from build123d import *

# Parameters (mm, degrees)
SKETCH1_R                                         = 16.7
SKETCH1_R_2                                       = 12.7
BOSS_EXTRUDE1_DEPTH                               = 10
SKETCH2_W                                         = 22.16607393
SKETCH2_H                                         = 10
SKETCH2_W_2                                       = 4
SKETCH2_H_2                                       = 30
BOSS_EXTRUDE2_DEPTH                               = 10
SKETCH4_W                                         = 8
SKETCH4_H                                         = 11.78611706
BOSS_EXTRUDE3_DEPTH                               = 10
FILLET3_R                                         = 1
CSK_FOR_6_FLAT_HEAD_MACHINE_SCREW_100_D           = 4.3053
CSK_FOR_6_FLAT_HEAD_MACHINE_SCREW_100_CSINK_D     = 7.0866
CSK_FOR_6_FLAT_HEAD_MACHINE_SCREW_100_CSINK_ANGLE = 100
INTERSECT3_START                                  = -42.1
INTERSECT3_OUTLINE_R                              = 2.15265
INTERSECT3_DEPTH                                  = 42.1


# Read off the part's stored shape, not the designer's step: CSK for #4 Flat Head Machine Screw (100)1, Intersect3
with BuildPart() as part:
    # Sketch1 → Boss-Extrude1 (new body)
    with BuildSketch(Plane.XY):
        Circle(SKETCH1_R)
        Circle(SKETCH1_R_2, mode=Mode.SUBTRACT)
    extrude(amount=BOSS_EXTRUDE1_DEPTH)

    # Sketch2 → Boss-Extrude2 (add)
    with BuildSketch(Plane(origin=(0, 0, 0), x_dir=(-1, 0, 0), z_dir=(0, 0, -1))):
        with Locations((27.016963035, 0)):
            Rectangle(SKETCH2_W, SKETCH2_H)
        with Locations((40.1, 0)):
            Rectangle(SKETCH2_W_2, SKETCH2_H_2)
    extrude(amount=-BOSS_EXTRUDE2_DEPTH)

    # Sketch4 → Boss-Extrude3 (add)
    with BuildSketch(Plane(origin=(0, 0, 0), x_dir=(-1, 0, 0), z_dir=(0, 0, -1))):
        with Locations((0, 22.10694147)):
            Rectangle(SKETCH4_W, SKETCH4_H)
    boss_extrude3 = extrude(amount=-BOSS_EXTRUDE3_DEPTH)

    # Mirror1: Boss-Extrude3 across plane
    add(boss_extrude3.mirror(Plane.ZX))

    # Fillet3
    fillet3_edges = [part.edges().sort_by_distance(p)[0] for p in [
        (-11.435827246, -12.170121413, 10),
        (-11.435827246, -12.170121413, 0),
        (-38.1, 10, 10),
        (-40.1, -15, 10),
        (-27.016963035, -5, 10),
        (-38.1, -10, 0),
        (-40.1, 15, 0),
        (-38.1, 10, 0),
        (-27.016963035, 5, 0),
        (-38.1, -10, 10),
        (-40.1, -15, 0),
        (-40.1, 15, 10),
        (-15.93392607, -5, 5),
        (-27.016963035, -5, 0),
        (-27.016963035, 5, 10),
        (-15.93392607, 5, 5),
        (-11.435827246, 12.170121413, 0),
        (-11.435827246, 12.170121413, 10),
        (-4, 22.10694147, 0),
        (0, 28, 0),
        (4, 22.10694147, 0),
        (0, 28, 10),
        (4, 28, 5),
        (4, 22.10694147, 10),
        (4, 16.21388294, 5),
        (-4, 16.21388294, 5),
        (-4, 22.10694147, 10),
        (-4, 28, 5),
        (16.7, 0, 0),
        (16.7, 0, 10),
        (-4, -16.21388294, 5),
        (-4, -22.10694147, 0),
        (-4, -28, 5),
        (0, -28, 0),
        (4, -28, 5),
        (4, -22.10694147, 0),
        (4, -16.21388294, 5),
        (-4, -22.10694147, 10),
        (0, -28, 10),
        (4, -22.10694147, 10),
    ]]
    fillet(fillet3_edges, radius=FILLET3_R)

    # CSK for _4 Flat Head Machine Screw _ 2 → CSK for #4 Flat Head Machine Screw (100)1 (revolve, cut)
    with BuildSketch(Plane(origin=(0, -9, 5), x_dir=(0, 1, 0), z_dir=(0, 0, -1))):
        Polygon((0, -42.1), (1.7272, -42.1), (1.7272, -39.048434313), (2.8575, -38.1), (0, -38.1), align=None)
    csk_for_4_flat_head_machine_screw_100 = revolve(axis=Axis((0, -9, 5), (1, 0, 0)), mode=Mode.SUBTRACT)

    # Mirror2: CSK for #4 Flat Head Machine Screw (100)1 across plane
    add(csk_for_4_flat_head_machine_screw_100.mirror(Plane.ZX), mode=Mode.SUBTRACT)

    # CSK for #6 Flat Head Machine Screw (100)5 (through all)
    with Locations(Plane.ZY.offset(4)):
        with Locations((5, -22)):
            csk_for_6_flat_head_machine_screw_100 = CounterSinkHole(CSK_FOR_6_FLAT_HEAD_MACHINE_SCREW_100_D / 2, CSK_FOR_6_FLAT_HEAD_MACHINE_SCREW_100_CSINK_D / 2, counter_sink_angle=CSK_FOR_6_FLAT_HEAD_MACHINE_SCREW_100_CSINK_ANGLE)

    # Mirror5: CSK for #6 Flat Head Machine Screw (100)5 across plane
    add(csk_for_6_flat_head_machine_screw_100.mirror(Plane.ZX), mode=Mode.SUBTRACT)

    # Intersect3 outline → Intersect3 (cut)
    with BuildSketch(Plane.YZ.offset(INTERSECT3_START)):
        with BuildLine():
            ThreePointArc((28, 9), (27.707106781, 9.707106781), (27, 10))
            Line((27, 10), (-27, 10))
            ThreePointArc((-27, 10), (-27.707106781, 9.707106781), (-28, 9))
            Line((-28, 9), (-28, 1))
            ThreePointArc((-28, 1), (-27.707106781, 0.292893219), (-27, 0))
            Line((-27, 0), (27, 0))
            ThreePointArc((27, 0), (27.707106781, 0.292893219), (28, 1))
            Line((28, 1), (28, 9))
        make_face()
        with Locations((22, 5)):
            Circle(INTERSECT3_OUTLINE_R, mode=Mode.SUBTRACT)
        with Locations((-22, 5)):
            Circle(INTERSECT3_OUTLINE_R, mode=Mode.SUBTRACT)
    extrude(amount=INTERSECT3_DEPTH, mode=Mode.SUBTRACT)


solid = part.part
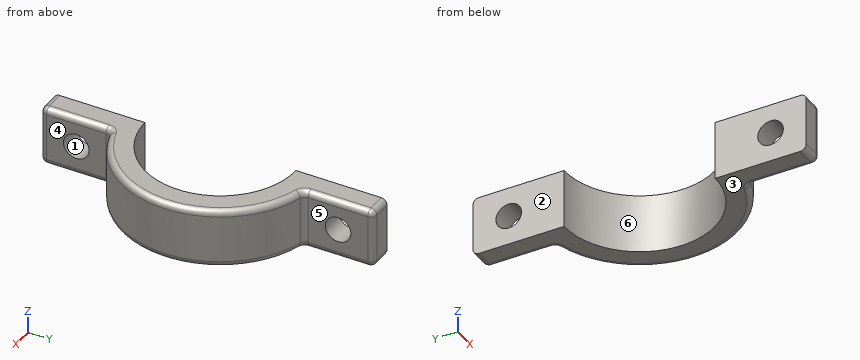
Build history of the part. All positions in model axes, mm. Face numbers are marked on the shaded views. A direction names the side the tool comes from. Give positions to 0.01 mm unless a question says otherwise; leave off trailing zeros. Write each loop counter-clockwise with the first axis right and the second up, starting at its lowest first coordinate (ties: lowest second). Pieces come first, ordered by that corner, then holes. Notation, with made-up numbers: (43.5, -17.75) - (93.5, -17.75) arc R9 ccw to (93.5, -6.75) - close; hole circle Ø2 at (-12, -29). An arc over 180 degrees is marked (long way). Use one line per item in the form item = value. Start each with the question number.
1. Band-saw the part on A-A on x = 1. Write the cut outline in (y, z), plus the area to 3 significant figures.
2. Band-saw the part on C-C on z = 5. Write the cut outline in (x, y).
3. Drop flat-ended pins along their axis: pin 1 Ø2 at (x, y) = (9, 16.5) entering from +Z; pin 2 Ø6 at (x, z) = (8.5, 4.5) entering from -Y; pin 3 Ø5 at (y, z) = (-21, 5) entering from +X; pin 4 Ø5 at (y, z) = (17, 8.5) entering from +X. Give the stop position or say it passes through.
4. Probe line 1 (Z direction, x = 1.2, y = -22); line 2 (Y direction, x = 1.3, z = 5); line 3 (X direction, y = 19, z = 7.5). List the from-to ranges inside material, lowest first. Write a range as [from, to].
5. Two-plate mould, pull along Z, no slides. Class the marked faces 1, 2 and 3: released by +Z, released by -Z, zero draft, split by the parting line, or undercut.
6. Band-saw the part on B-B on y = -22. Write the cut outline in (x, z).
7. 3-axis set-ups, long thin cutter, end or side, ignore diameter. For the marked faces 4, 5 and 6: which of +Z, -Z, +X, -X, +Y, -Y reach the whole face in a straight line?
Conclusion:
q1.outline = (-28, 1) arc R1 ccw to (-27, 0) - (-12.66, 0) - (-12.66, 10) - (-27, 10) arc R1 ccw to (-28, 9) - close; (12.66, 0) - (27, 0) arc R1 ccw to (28, 1) - (28, 9) arc R1 ccw to (27, 10) - (12.66, 10) - close; hole circle Ø4.31 at (-22, 5); hole circle Ø4.31 at (22, 5)
q1.area = 277 mm²
q2.outline = (0, -28) - (3, -28) arc R1 ccw to (4, -27) - (4, -24.15) - (0, -24.15) - close; (0, -19.85) - (4, -19.85) - (4, -16.98) arc R1 cw to (4.72, -16.02) arc R16.7 ccw to (4.72, 16.02) arc R1 cw to (4, 16.98) - (4, 19.85) - (0, 19.85) - (0, 12.7) arc R12.7 cw to (0, -12.7) - close; (0, 24.15) - (4, 24.15) - (4, 27) arc R1 ccw to (3, 28) - (0, 28) - close
q3.pin_1 = through
q3.pin_2 = -15.77
q3.pin_3 = 4
q3.pin_4 = 8.28
q4.line_1 = [0, 2.85], [7.15, 10]
q4.line_2 = [-28, -24.15], [-19.85, -12.63], [12.63, 19.85], [24.15, 28]
q4.line_3 = [0, 4]
q5.face_1 = undercut
q5.face_2 = zero draft
q5.face_3 = released by -Z
q6.outline = (0, 0) - (3, 0) arc R1 ccw to (4, 1) - (4, 2.85) - (0, 2.85) - close; (0, 7.15) - (4, 7.15) - (4, 9) arc R1 ccw to (3, 10) - (0, 10) - close
q7.face_4 = +Z, -Z, +X, -Y
q7.face_5 = +Z, -Z, +X, +Y
q7.face_6 = +Z, -Z, -X
